```python
from build123d import *

# Parameters (mm, degrees)
ESQUISSE1_R             = 1.7
BOSS_EXTRU_1_DEPTH      = 3
ESQUISSE2_R             = 5.2
BOSS_EXTRU_2_DEPTH      = 3
BOSS_EXTRU_2_DEPTH_BACK = 3
ESQUISSE5_W             = 129.390100882
ESQUISSE5_H             = 110.068207502
ENL_V_MAT_EXTRU_2_DEPTH = 1
ESQUISSE6_R             = 1.5
ENL_V_MAT_EXTRU_3_DEPTH = 8
ESQUISSE7_W             = 14.610679854
ESQUISSE7_H             = 62.75
ENL_V_MAT_EXTRU_4_DEPTH = 8
BOSS_EXTRU_3_DEPTH      = 7
BOSS_EXTRU_4_DEPTH      = 7


with BuildPart() as part:
    # Esquisse1 → Boss.-Extru.1 (new body)
    with BuildSketch(Plane.XY):
        with BuildLine():
            Line((-117.680084405, 66.939310237), (-117.680084405, 59.695120061))
            ThreePointArc((-117.680084405, 59.695120061), (-116.069171702, 55.806032765), (-112.180084405, 54.195120061))
            Line((-112.180084405, 54.195120061), (-105.294175096, 54.195120061))
            ThreePointArc((-105.294175096, 54.195120061), (-101.4050878, 52.584207358), (-99.794175096, 48.695120061))
            Line((-99.794175096, 48.695120061), (-99.794175096, 35.930823665))
            ThreePointArc((-99.794175096, 35.930823665), (-101.4050878, 32.041736368), (-105.294175096, 30.430823665))
            Line((-105.294175096, 30.430823665), (-112.180084405, 30.430823665))
            ThreePointArc((-112.180084405, 30.430823665), (-116.069171702, 28.819910961), (-117.680084405, 24.930823665))
            Line((-117.680084405, 24.930823665), (-117.680084405, 23.910007682))
            ThreePointArc((-117.680084405, 23.910007682), (-116.069171702, 20.020920385), (-112.180084405, 18.410007682))
            Line((-112.180084405, 18.410007682), (-105.294175096, 18.410007682))
            ThreePointArc((-105.294175096, 18.410007682), (-101.4050878, 16.799094979), (-99.794175096, 12.910007682))
            Line((-99.794175096, 12.910007682), (-99.794175096, 1.692208933))
            ThreePointArc((-99.794175096, 1.692208933), (-101.4050878, -2.196878364), (-105.294175096, -3.807791067))
            Line((-105.294175096, -3.807791067), (-113.390601299, -3.807791067))
            ThreePointArc((-113.390601299, -3.807791067), (-117.279688595, -5.418703771), (-118.890601299, -9.307791067))
            Line((-118.890601299, -9.307791067), (-118.890601299, -18.42196685))
            ThreePointArc((-118.890601299, -18.42196685), (-117.279688595, -22.311054147), (-113.390601299, -23.92196685))
            Line((-113.390601299, -23.92196685), (-52.866544484, -23.92196685))
            ThreePointArc((-52.866544484, -23.92196685), (-48.977457187, -22.311054147), (-47.366544484, -18.42196685))
            Line((-47.366544484, -18.42196685), (-47.366544484, -9.307791067))
            ThreePointArc((-47.366544484, -9.307791067), (-48.977457187, -5.418703771), (-52.866544484, -3.807791067))
            Line((-52.866544484, -3.807791067), (-77.986378892, -3.807791067))
            ThreePointArc((-77.986378892, -3.807791067), (-81.875466189, -2.196878364), (-83.486378892, 1.692208933))
            Line((-83.486378892, 1.692208933), (-83.486378892, 12.910007682))
            ThreePointArc((-83.486378892, 12.910007682), (-81.875466189, 16.799094979), (-77.986378892, 18.410007682))
            Line((-77.986378892, 18.410007682), (-69.856378892, 18.410007682))
            ThreePointArc((-69.856378892, 18.410007682), (-65.967291596, 20.020920385), (-64.356378892, 23.910007682))
            Line((-64.356378892, 23.910007682), (-64.356378892, 24.930823665))
            ThreePointArc((-64.356378892, 24.930823665), (-65.967291596, 28.819910961), (-69.856378892, 30.430823665))
            Line((-69.856378892, 30.430823665), (-77.986378892, 30.430823665))
            ThreePointArc((-77.986378892, 30.430823665), (-81.875466189, 32.041736368), (-83.486378892, 35.930823665))
            Line((-83.486378892, 35.930823665), (-83.486378892, 55.219310237))
            ThreePointArc((-83.486378892, 55.219310237), (-81.875466189, 59.108397534), (-77.986378892, 60.719310237))
            Line((-77.986378892, 60.719310237), (-54.190366806, 60.719310237))
            ThreePointArc((-54.190366806, 60.719310237), (-50.30127951, 62.330222941), (-48.690366806, 66.219310237))
            Line((-48.690366806, 66.219310237), (-48.690366806, 67.219310237))
            ThreePointArc((-48.690366806, 67.219310237), (-50.30127951, 71.108397534), (-54.190366806, 72.719310237))
            Line((-54.190366806, 72.719310237), (-112.180084405, 72.719310237))
            ThreePointArc((-112.180084405, 72.719310237), (-116.069171702, 71.108397534), (-117.680084405, 67.219310237))
            Line((-117.680084405, 67.219310237), (-117.680084405, 66.939310237))
        make_face()
        with Locations((-59.266378892, -15.663707737)):
            Circle(ESQUISSE1_R, mode=Mode.SUBTRACT)
        with Locations((-59.266378892, 66.939310237)):
            Circle(ESQUISSE1_R, mode=Mode.SUBTRACT)
        with Locations((-91.856378892, 36.719310237)):
            Circle(ESQUISSE1_R, mode=Mode.SUBTRACT)
        with Locations((-107.466378892, -14.520689763)):
            Circle(ESQUISSE1_R, mode=Mode.SUBTRACT)
        with Locations((-107.466378892, 60.719310237)):
            Circle(ESQUISSE1_R, mode=Mode.SUBTRACT)
        with BuildLine():
            Line((-111.390601299, 21.460065469), (-70.086378892, 21.460065469))
            ThreePointArc((-70.086378892, 21.460065469), (-68.67216533, 22.045851906), (-68.086378892, 23.460065469))
            Line((-68.086378892, 23.460065469), (-68.086378892, 24.842520386))
            ThreePointArc((-68.086378892, 24.842520386), (-68.67216533, 26.256733949), (-70.086378892, 26.842520386))
            Line((-70.086378892, 26.842520386), (-111.390601299, 26.842520386))
            ThreePointArc((-111.390601299, 26.842520386), (-112.804814861, 26.256733949), (-113.390601299, 24.842520386))
            Line((-113.390601299, 24.842520386), (-113.390601299, 23.460065469))
            ThreePointArc((-113.390601299, 23.460065469), (-112.804814861, 22.045851906), (-111.390601299, 21.460065469))
        make_face(mode=Mode.SUBTRACT)
    extrude(amount=BOSS_EXTRU_1_DEPTH)

    # Esquisse2 → Boss.-Extru.2 (add, two sides)
    with BuildSketch(Plane(origin=(0, 0, 0), x_dir=(-1, 0, 0), z_dir=(0, 0, -1))) as boss_extru_2_sk:
        with BuildLine():
            Line((118.890601299, -9.969506719), (130.584615963, -9.880075131))
            ThreePointArc((130.584615963, -9.880075131), (134.095405897, -8.402210456), (135.546378892, -4.880221341))
            Line((135.546378892, -4.880221341), (135.546378892, 5.415623015))
            ThreePointArc((135.546378892, 5.415623015), (136.425058549, 7.536943358), (138.546378892, 8.415623015))
            Line((138.546378892, 8.415623015), (145.752654566, 8.415623015))
            ThreePointArc((145.752654566, 8.415623015), (147.87397491, 9.294302671), (148.752654566, 11.415623015))
            Line((148.752654566, 11.415623015), (148.752654566, 38.179170847))
            ThreePointArc((148.752654566, 38.179170847), (147.87397491, 40.300491191), (145.752654566, 41.179170847))
            Line((145.752654566, 41.179170847), (138.546378892, 41.179170847))
            ThreePointArc((138.546378892, 41.179170847), (136.425058549, 42.057850504), (135.546378892, 44.179170847))
            Line((135.546378892, 44.179170847), (135.546378892, 52.099902349))
            ThreePointArc((135.546378892, 52.099902349), (134.081912798, 55.635436255), (130.546378892, 57.099902349))
            Line((130.546378892, 57.099902349), (117.680084405, 57.099902349))
            Line((117.680084405, 57.099902349), (117.680084405, 72.719310237))
            Line((117.680084405, 72.719310237), (48.690366806, 72.719310237))
            Line((48.690366806, 72.719310237), (48.690366806, 60.719310237))
            Line((48.690366806, 60.719310237), (48.690366806, 57.099902349))
            Line((48.690366806, 57.099902349), (40.256901013, 57.099902349))
            ThreePointArc((40.256901013, 57.099902349), (37.428473888, 55.928329474), (36.256901013, 53.099902349))
            Line((36.256901013, 53.099902349), (36.256901013, 47.456292263))
            Line((36.256901013, 47.456292263), (39.346378892, 47.456292263))
            ThreePointArc((39.346378892, 47.456292263), (41.396631424, 52.406039732), (46.346378892, 54.456292263))
            Line((46.346378892, 54.456292263), (126.246378892, 54.456292263))
            ThreePointArc((126.246378892, 54.456292263), (131.196126361, 52.406039732), (133.246378892, 47.456292263))
            Line((133.246378892, 47.456292263), (133.246378892, 40.977229779))
            ThreePointArc((133.246378892, 40.977229779), (134.125058549, 38.855909436), (136.246378892, 37.977229779))
            Line((136.246378892, 37.977229779), (142.162261637, 37.977229779))
            ThreePointArc((142.162261637, 37.977229779), (144.28358198, 37.098550123), (145.162261637, 34.977229779))
            Line((145.162261637, 34.977229779), (145.162261637, 14.363062522))
            ThreePointArc((145.162261637, 14.363062522), (144.28358198, 12.241742179), (142.162261637, 11.363062522))
            Line((142.162261637, 11.363062522), (136.246378892, 11.363062522))
            ThreePointArc((136.246378892, 11.363062522), (134.125058549, 10.484382866), (133.246378892, 8.363062522))
            Line((133.246378892, 8.363062522), (133.246378892, -1.293707737))
            ThreePointArc((133.246378892, -1.293707737), (131.196126361, -6.243455205), (126.246378892, -8.293707737))
            Line((126.246378892, -8.293707737), (46.346378892, -8.293707737))
            ThreePointArc((46.346378892, -8.293707737), (41.396631424, -6.243455205), (39.346378892, -1.293707737))
            Line((39.346378892, -1.293707737), (36.248203357, -1.293707737))
            Line((36.248203357, -1.293707737), (36.248203357, -6.64542392))
            ThreePointArc((36.248203357, -6.64542392), (37.432020164, -9.486042202), (40.282759469, -10.645274652))
            Line((40.282759469, -10.645274652), (47.366544484, -10.58407535))
            Line((47.366544484, -10.58407535), (47.366544484, -23.92196685))
            Line((47.366544484, -23.92196685), (118.890601299, -23.92196685))
            Line((118.890601299, -23.92196685), (118.890601299, -9.969506719))
        make_face()
        with Locations((59.266378892, -15.663707737)):
            Circle(ESQUISSE2_R, mode=Mode.SUBTRACT)
        with Locations((107.466378892, -14.520689763)):
            Circle(ESQUISSE2_R, mode=Mode.SUBTRACT)
        with Locations((107.466378892, 60.719310237)):
            Circle(ESQUISSE2_R, mode=Mode.SUBTRACT)
        with Locations((59.266378892, 66.939310237)):
            Circle(ESQUISSE2_R, mode=Mode.SUBTRACT)
    extrude(amount=BOSS_EXTRU_2_DEPTH)
    extrude(boss_extru_2_sk.sketch, amount=-BOSS_EXTRU_2_DEPTH_BACK)

    # Esquisse5 → Enl_v. mat.-Extru.2 (cut)
    with BuildSketch(Plane.XY.offset(3)):
        with Locations((-91.695706627, 24.836368366)):
            Rectangle(ESQUISSE5_W, ESQUISSE5_H)
    extrude(amount=-ENL_V_MAT_EXTRU_2_DEPTH, mode=Mode.SUBTRACT)

    # Esquisse6 → Enl_v. mat.-Extru.3 (cut)
    with BuildSketch(Plane.XY.offset(2)):
        with Locations((-69.623492164, 64.727424081)):
            Circle(ESQUISSE6_R)
        with Locations((-83.623492164, 64.727424081)):
            Circle(ESQUISSE6_R)
    extrude(amount=-ENL_V_MAT_EXTRU_3_DEPTH, mode=Mode.SUBTRACT)

    # Esquisse7 → Enl_v. mat.-Extru.4 (cut)
    with BuildSketch(Plane(origin=(0, 0, 0), x_dir=(-1, 0, 0), z_dir=(0, 0, -1))):
        with Locations((42.567758063, 23.081292263)):
            Rectangle(ESQUISSE7_W, ESQUISSE7_H)
    extrude(amount=ENL_V_MAT_EXTRU_4_DEPTH, mode=Mode.SUBTRACT)

    # Esquisse9 → Boss.-Extru.3 (add)
    with BuildSketch(Plane(origin=(0, -1.293707737, 0), x_dir=(1, 0, 0), z_dir=(0, 1, 0))):
        Polygon((-39.346378892, -2), (-39.346378892, 0.886005049), (-36.248203357, 0), (-36.248203357, -2), align=None)
    extrude(amount=-BOSS_EXTRU_3_DEPTH)

    # Esquisse10 → Boss.-Extru.4 (add)
    with BuildSketch(Plane.XZ.offset(-47.456292263)):
        Polygon((-39.346378892, 2), (-39.346378892, -0.873043126), (-36.256901013, 0), (-36.256901013, 2), align=None)
    extrude(amount=-BOSS_EXTRU_4_DEPTH)


solid = part.part
```
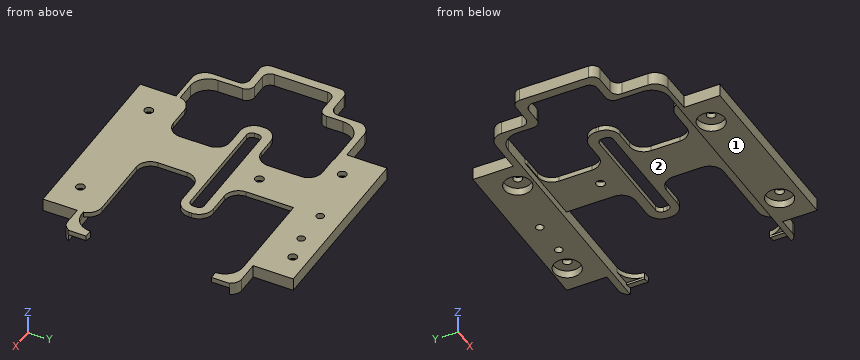
Design review of the part built by this model. Coordinates are the model's own, in mm. Face numbers are marked on the shaded views. Coordinates: 2 decimals unless noted, no trailing zeros. Order: outer loops, then holes, each group sorted by start corner. A loop starts at its lowest first (then second) coordinate and runs counter-clockwise, first axis right, second up. Notation, with made-up numbers: M -1,-6 L 25,-6 A24 ccw 25,10 Z; hole C 61.5,70.5 d9. An arc over 180 degrees is marked long. Answer as a JSON object with one key per item and string values. Group by question number.
1) Add section A-A, the plane x = -95.5. Write out the cut boundary in (y, z).
2) Add section D-D, the plane y = 17. Write out the cut boundary in (x, z).
3) Add section B-B, the plane y = 7. Write out the cut boundary in (x, z).
4) For pin 1 (1.5 mm diameter, centred on y = 46, z = -0.5, fed in from +X); pin 2 (1.5 mm diameter, centred on y = 2.5, z = -0.5, fed in from -X); pin 3 (1.1 mm diameter, centred on y = 24.5, z = 1, fed in from +X); pin 4 (3.5 mm diameter, centred on x = -43.5, y = 51.5, fed in from -Z), all flat-tipped, find the tip position at first contact; note any pin that passes through.
5) Add section C-C, the plane z = 1.15. Count the separate pieces of the cut face and the enclosed holes in it, then the cut area to 3 significant figures.
6) Wall thickness on L1, parallel to Y at x = -53, z = -1.55; L2, parallel to Y at x = -85, z = 0.1; L3, parallel to X at y = -18, z = -2.55: over which ranges is each line inside the solid? List them lowest first.
7) Mouldability with a two-part tool opening along X and no side actions: class the marked faces 1 and 2 as pulls with the +X half, pulls with the -X half, needs draft (parallel to the pull), parting line crosses it, or undercut.
Computed values:
{
 "1": {"outline": "M -23.92,-3 L -8.29,-3 L -8.29,0 L 21.46,0 L 21.46,2 L -23.92,2 Z; M 26.84,0 L 54.46,0 L 54.46,-3 L 72.72,-3 L 72.72,2 L 26.84,2 Z"},
 "2": {"outline": "M -148.75,-3 L -145.16,-3 L -145.16,2 L -148.75,2 Z; M -101.62,0 L -81.66,0 L -81.66,2 L -101.62,2 Z"},
 "3": {"outline": "M -136,-3 L -133.25,-3 L -133.25,2 L -136,2 Z; M -99.79,0 L -83.49,0 L -83.49,2 L -99.79,2 Z"},
 "4": {"pin 1": "stops at x = -83.49", "pin 2": "stops at x = -135.55", "pin 3": "stops at x = -64.36", "pin 4": "passes through"},
 "5": {"separate pieces": "1", "enclosed holes": "9", "area": "4,260 mm^2"},
 "6": {"L1": "y = -23.92 to -8.29, 54.46 to 72.72", "L2": "y = -23.92 to 21.46, 26.84 to 64.13, 65.32 to 72.72", "L3": "x = -118.89 to -111.33, -103.6 to -63.91, -54.62 to -47.37"},
 "7": {"face 1": "needs draft", "face 2": "undercut"}
}
